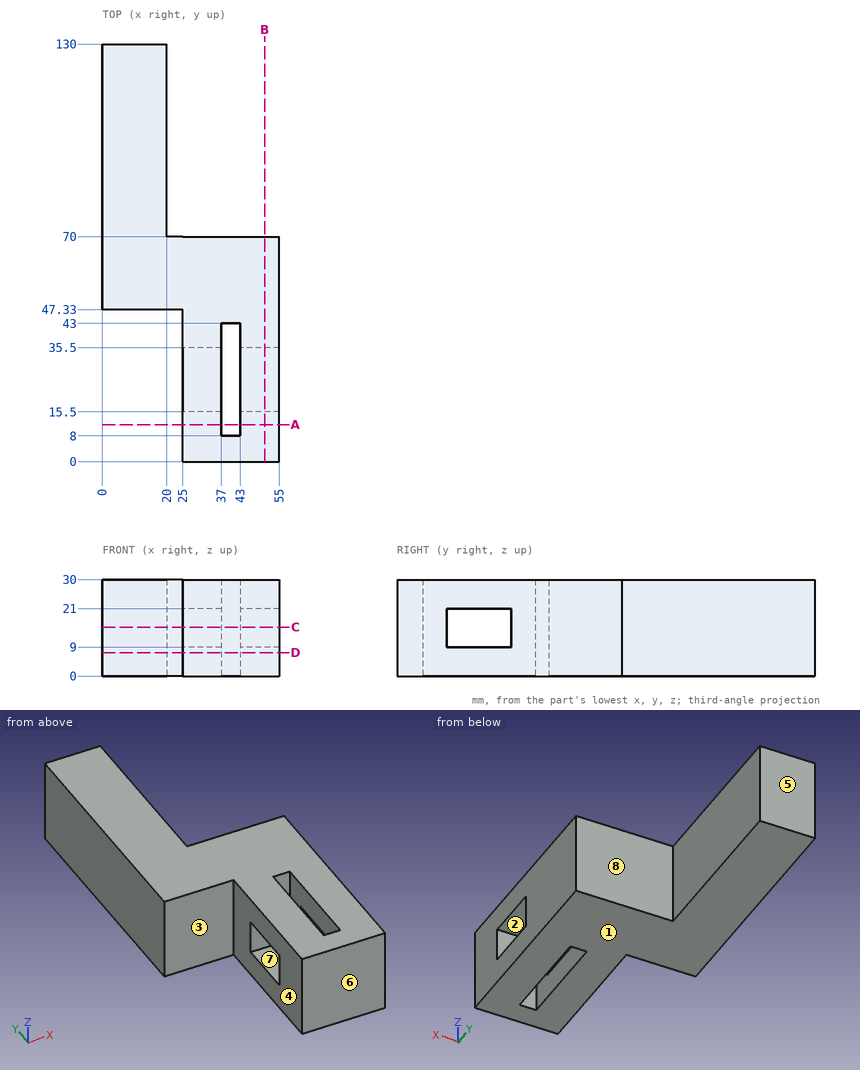
Study the drawing (mm; zero at the part's minimum x, y, z) and answer. A direction names the side the tool comes from. Coordinates: 2 decimals unless noted, no trailing zeros. Write each loop counter-clockwise with the first axis right and the second up, starting at its lowest first coordinate (ties: lowest second). Pieces come first, ordered by that corner, then holes. Notation, with made-up numbers: M 75,-31.5 L 88,-31.5 A23 ccw 88,-9.5 Z; hole C 0,60.5 d2. An arc over 180 degrees is marked long. Write each question's results on one line, items separated by ' | '.
Item 1: Which of the six approach directions +Z, -Z, +X, -X, +Y, -Y give full straight-line access (tool end or side, diameter ignored) to the marked faces 4, 5, 6, 7 and 8?
Answer below:
face 4: +Z, -Z, -X, -Y | face 5: +Z, -Z, +X, -X, +Y | face 6: +Z, -Z, +X, -X, -Y | face 7: +X, -X | face 8: +Z, -Z, +X, +Y
Item 2: The part is cut by section D-D on z = 7.25. Determine the outline of the cut face in (x, y), and give its area (3 significant figures).
Answer below:
outline: M 0,47.33 L 25,47.33 L 25,0 L 55,0 L 55,70 L 20,70 L 20,130 L 0,130 Z; hole M 37,8 L 43,8 L 43,43 L 37,43 Z | area: 3,660 mm2
Item 3: The part is cut by section B-B on x = 50.5. Determine the outline of the cut face in (y, z).
Answer below:
outline: M 0,0 L 70,0 L 70,30 L 0,30 Z; hole M 15.5,9 L 35.5,9 L 35.5,21 L 15.5,21 Z
Item 4: For a pull along Y with two mould halves and no side action, classify the marked faces 1, 2 and 3 as released by +Y, released by -Y, zero draft, split by the parting line, or undercut.
Answer below:
face 1: zero draft | face 2: undercut | face 3: released by -Y
Item 5: The part is cut by section C-C on z = 15.25. Determine the outline of the cut face in (x, y), and give its area (3 significant figures).
Answer below:
outline: M 0,47.33 L 25,47.33 L 25,35.5 L 37,35.5 L 37,43 L 43,43 L 43,35.5 L 55,35.5 L 55,70 L 20,70 L 20,130 L 0,130 Z; M 25,0 L 55,0 L 55,15.5 L 43,15.5 L 43,8 L 37,8 L 37,15.5 L 25,15.5 Z | area: 3,180 mm2
Item 6: Given P1, Ø8, axis at y = 35.5, z = 26.5, coming from the -X side; P2, Ø1.5, axis at x = 36, z = 26, coming from the +Y side; P3, Ø12.5, axis at x = 14.5, z = 20.5, coming from the -Y side, each flat-ended and moving along its own axis, determine where each tip first touches the part or whether it passes through.
Answer below:
P1: x = 25 | P2: y = 70 | P3: y = 47.33
Item 7: Consider probe 1 along X at (y, z) = (29, 6); probe 2 along Y at (x, z) = (41.5, 22.5); probe 3 along Y at (x, z) = (45, 10.75). Determine where each line is inside the solid, lowest interval first. Write a range as [from, to].
Answer below:
probe 1: [25, 37], [43, 55] | probe 2: [0, 8], [43, 70] | probe 3: [0, 15.5], [35.5, 70]
Item 8: The part is cut by section A-A on y = 11.5. Determine the outline of the cut face in (x, z), and give its area (3 significant figures).
Answer below:
outline: M 25,0 L 37,0 L 37,30 L 25,30 Z; M 43,0 L 55,0 L 55,30 L 43,30 Z | area: 720 mm2
